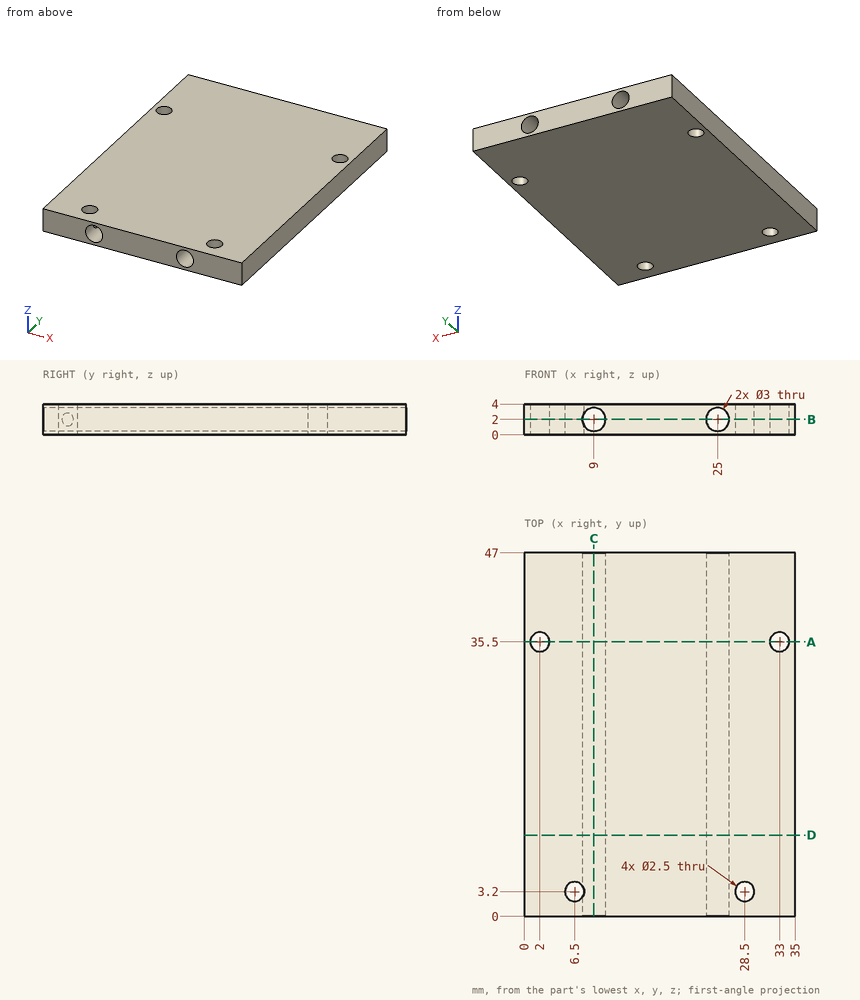
The drawing under review shows one solid part. Ordinate dimensions are in mm from its lowest x, y, z. Give positions to 0.01 mm unless a question says otherwise; leave off trailing zeros. Loops run counter-clockwise (first coordinate to the right, second up) from the corner with the lowest first, then second, coordinate; pieces in that order, holes last. Notation, with made-up numbers: M 8,49 L 12,49 A34 ccw 12,88 Z; hole C 77,-40 d5. An arc over 180 degrees is marked long. Return JSON: item names as keys, results as strings. Group by question number.
Item 1: We need section B-B (z = 2). Give the boundary of the cut face in (x, y), and give its area (3 significant figures).
Item 2: Insertion check: pin 1 Ø4 at (x, y) = (6.5, 3.2) entering from +Z. The pin has a flat end and moves straight along its axis. Give the tip position at first contact, or say it passes through.
Item 3: We need section C-C (x = 9). Give the boundary of the cut face in (y, z).
Item 4: We need section D-D (y = 10.5). Give the boundary of the cut face in (x, z).
Item 5: For probe 1 along X at (y, z) = (21, 2.15); probe 2 along Z at (x, y) = (9, 25); probe 3 along Y at (x, z) = (6.5, 0.9), list the stretches that pass through material, from the lowest coordinate up.
Item 6: We need section A-A (y = 35.5). Give the boundary of the cut face in (x, z).
Output:
{
 "1": {"outline": "M 0,0 L 7.5,0 L 7.5,2.45 A1.25 cw long 7.5,3.95 L 7.5,47 L 0,47 Z; M 10.5,0 L 23.5,0 L 23.5,47 L 10.5,47 Z; M 26.5,0 L 35,0 L 35,47 L 26.5,47 Z; hole C 2,35.5 d2.5; hole C 28.5,3.2 d2.5; hole C 33,35.5 d2.5", "area": "1,340 mm^2"},
 "2": {"pin 1": "stops at z = 4"},
 "3": {"outline": "M 0,0 L 47,0 L 47,0.5 L 0,0.5 Z; M 0,3.5 L 47,3.5 L 47,4 L 0,4 Z"},
 "4": {"outline": "M 0,0 L 35,0 L 35,4 L 0,4 Z; hole C 9,2 d3; hole C 25,2 d3"},
 "5": {"probe 1": "x = 0 to 7.51, 10.49 to 23.51, 26.49 to 35", "probe 2": "z = 0 to 0.5, 3.5 to 4", "probe 3": "y = 0 to 1.95, 4.45 to 47"},
 "6": {"outline": "M 0,0 L 0.75,0 L 0.75,4 L 0,4 Z; M 3.25,0 L 31.75,0 L 31.75,4 L 3.25,4 Z; M 34.25,0 L 35,0 L 35,4 L 34.25,4 Z; hole C 9,2 d3; hole C 25,2 d3"}
}
